Source: CAD feature listing. Evaluate the final solid. Frame: model axes, mm. Face numbers are marked on the shaded views. A direction names the side the tool comes from. Round coordinates to 2 decimals unless told otherwise and drop trailing zeros. Order: outer loops, then holes, each group sorted by start corner. A loop starts at its lowest first (then second) coordinate and runs counter-clockwise, first axis right, second up. Notation, with made-up numbers: M 78,-38.5 L 103,-38.5 A19 cw 103,-22.5 Z; hole C 36.25,69 d7. An arc over 180 degrees is marked long. Answer as CSV lines item,"result". Start each with the question number.
Item 1: Set-up query: the marked faces 1 and 2. Return all of +Z, -Z, +X, -X, +Y, -Y with unobstructed straight access to the full face (end or side cutting, diameter ignored); none if empty.
Item 2: Line query: line 1 (Y direction, x = 35.5, z = 176); line 2 (Z direction, x = -17.5, y = -1.15); line 3 (X direction, y = 36, z = 165). Output: solid intervals per line, ascending. Write a range as [from, to].
Item 3: First-contact query: P1, Ø1.3, axis at y = 52.5, z = 4, coming from the +X side; P2, Ø4, axis at x = -23, z = 50, coming from the +Y side. Flat tips, straight axial feed; report the tip coordinate or a pass-through.
Item 4: Section query C-C on x = 31.5. Return the cut outline in (y, z), plus the area to 3 significant figures.
Item 5: Section query A-A on y = 65. Return the cut outline in (x, z).
Item 6: Section query B-B on z = 151.5. Return the cut outline in (x, y), plus the area to 3 significant figures.
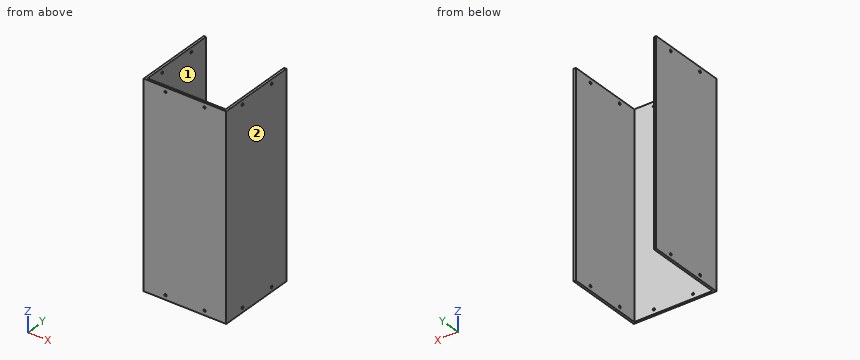
from build123d import *

# Parameters (mm, degrees)
EXTRUDE_3_DEPTH     = 180
SKETCH_3_R          = 1.1
CUT_EXTRUDE_1_DEPTH = 207.823596333
SKETCH_4_R          = 1
CUT_EXTRUDE_2_DEPTH = 197.644349016


with BuildPart() as part:
    # 草图2 → 凸台-拉伸3 (new body)
    with BuildSketch(Plane.XY):
        Polygon((-35, 0), (35, 0), (35, 70), (37, 70), (37, -2), (-37, -2), (-37, 70), (-35, 70), align=None)
    extrude(amount=EXTRUDE_3_DEPTH)

    # 草图3 → 切除-拉伸1 (cut, through all)
    with BuildSketch(Plane(origin=(37, 0, 0), x_dir=(0, 0, -1), z_dir=(1, 0, 0))):
        with Locations((-4, 52.5)):
            Circle(SKETCH_3_R)
        with Locations((-4, 17.5)):
            Circle(SKETCH_3_R)
    cut_extrude_1 = extrude(amount=-CUT_EXTRUDE_1_DEPTH, mode=Mode.SUBTRACT)

    # 镜向1: 切除-拉伸1 across plane
    add(cut_extrude_1.mirror(Plane(origin=(0, 0, 90), x_dir=(1, 0, 0), z_dir=(0, 0, -1))), mode=Mode.SUBTRACT)

    # 草图4 → 切除-拉伸2 (cut, through all)
    with BuildSketch(Plane(origin=(0, 0, 0), x_dir=(1, 0, 0), z_dir=(0, 1, 0))):
        with Locations(Location((-17.5, -4, 0), (0, 0, 180))):
            Circle(SKETCH_4_R)
        with Locations((17.5, -4)):
            Circle(SKETCH_4_R)
        with Locations((-17.5, -176)):
            Circle(SKETCH_4_R)
        with Locations(Location((17.5, -176, 0), (0, 0, 180))):
            Circle(SKETCH_4_R)
    extrude(amount=-CUT_EXTRUDE_2_DEPTH, mode=Mode.SUBTRACT)


solid = part.part
Results:
1,face 1,"+Z, -Z, +Y"
1,face 2,"+Z, -Z, +X, +Y, -Y"
2,line 1,"[-2, 16.4], [18.6, 51.4], [53.6, 70]"
2,line 2,"[0, 3], [5, 175], [177, 180]"
2,line 3,"[-37, -35], [35, 37]"
3,P1,"through"
3,P2,"y = 0"
4,outline,"M -2,0 L 0,0 L 0,180 L -2,180 Z"
4,area,"360 mm^2"
5,outline,"M -37,0 L -35,0 L -35,180 L -37,180 Z; M 35,0 L 37,0 L 37,180 L 35,180 Z"
6,outline,"M -37,-2 L 37,-2 L 37,70 L 35,70 L 35,0 L -35,0 L -35,70 L -37,70 Z"
6,area,"428 mm^2"
